Can you work these out from the model? Positions are in its coordinate system, mm. Face numbers are marked on the shaded views. A direction names the side the tool comes from. Round coordinates to 2 decimals unless told otherwise and drop trailing zeros. Write each loop counter-clockwise with the first axis right and the second up, starting at its lowest first coordinate (ties: lowest second). Pieces come first, ordered by that corner, then holes. Notation, with made-up numbers: (-29.75, 51.5) -> (15.25, 51.5) arc R34 ccw to (15.25, 81.5) -> close; hole circle Ø6 at (-10, 7). An arc over 180 degrees is marked (long way). Write item = value, one per line. Start each with the question number.
1) Imagine slicing it at B-B, the plane x = 9. Please give me the cut outline in (y, z), then the cut area to 3 significant figures.
2) I'm going to push flat-ended pins straight in: pin 1 (4 mm diameter, centred on x = -4.5, z = -7.79, fed in from +Y); pin 2 (6 mm diameter, centred on x = 4.5, z = 7.79, fed in from -Y); pin 3 (1 mm diameter, centred on x = 2.5, y = 1.5, fed in from +Z); pin 4 (1.5 mm diameter, centred on y = 3.5, z = -3, fed in from -X). Where does each tip first touch, or does it pass through?
3) Imagine slicing it at A-A, the plane z = 0. Please give me the cut outline in (x, y), then the cut area to 3 significant figures.
4) For the marked faces 1 and 2, which set-ups out of +Z, -Z, +X, -X, +Y, -Y let a thin tool reach every point of the face, with its end or its side?
5) Imagine slicing it at C-C, the plane x = -5. Please give me the cut outline in (y, z).
6) Imagine slicing it at D-D, the plane y = 2.95. Please give me the cut outline in (x, z).
7) Thinking about a two-plate mould opening in Z: for the marked faces 3, 4 and 5, which applies, +Z half, -Z half, draft (parallel to the pull), parting line (faces both ways), or undercut?
8) If I drill on line 1 (X direction, y = 2.8, z = 0); line 2 (Z direction, x = -4.5, y = 3.2); line 3 (X direction, y = 2.9, z = -2.25), over which ranges is the centre line in solid material (lowest first)?
from build123d import *

# Parameters (mm, degrees)
SKETCH_1_R          = 14
EXTRUDE_1_DEPTH     = 2
SKETCH_2_R          = 12.5
EXTRUDE_2_DEPTH     = 3
SKETCH_3_R          = 1.6
CUT_EXTRUDE_1_DEPTH = 6
SKETCH_4_R          = 3
CUT_EXTRUDE_2_DEPTH = 3.3
SKETCH_5_R          = 1.95
CUT_EXTRUDE_3_DEPTH = 3.2
CHAMFER_1_SIZE      = 0.5
SKETCH_6_R          = 3.5
CUT_EXTRUDE_4_DEPTH = 6


with BuildPart() as part:
    # 草图1 → 凸台-拉伸1 (new body)
    with BuildSketch(Plane(origin=(0, 0, 0), x_dir=(1, 0, 0), z_dir=(0, 1, 0))):
        Circle(SKETCH_1_R)
    extrude(amount=EXTRUDE_1_DEPTH)

    # 草图2 → 凸台-拉伸2 (add)
    with BuildSketch(Plane(origin=(0, 2, 0), x_dir=(1, 0, 0), z_dir=(0, 1, 0))):
        Circle(SKETCH_2_R)
    extrude(amount=EXTRUDE_2_DEPTH)

    # 草图3 → 切除-拉伸1 (cut, through all)
    with BuildSketch(Plane(origin=(0, 5, 0), x_dir=(1, 0, 0), z_dir=(0, 1, 0))):
        with Locations((9, 0)):
            Circle(SKETCH_3_R)
        with Locations((-4.5, -7.794228634)):
            Circle(SKETCH_3_R)
        with Locations((-4.5, 7.794228634)):
            Circle(SKETCH_3_R)
    extrude(amount=-CUT_EXTRUDE_1_DEPTH, mode=Mode.SUBTRACT)

    # 草图4 → 切除-拉伸2 (cut)
    with BuildSketch(Plane(origin=(0, 5, 0), x_dir=(1, 0, 0), z_dir=(0, 1, 0))):
        with Locations((9, 0)):
            Circle(SKETCH_4_R)
        with Locations((-4.5, 7.794228634)):
            Circle(SKETCH_4_R)
        with Locations((-4.5, -7.794228634)):
            Circle(SKETCH_4_R)
    extrude(amount=-CUT_EXTRUDE_2_DEPTH, mode=Mode.SUBTRACT)

    # 草图5 → 切除-拉伸3 (cut)
    with BuildSketch(Plane(origin=(0, 5, 0), x_dir=(1, 0, 0), z_dir=(0, 1, 0))):
        with Locations((4.5, 7.794228634)):
            Circle(SKETCH_5_R)
        with Locations((4.5, -7.794228634)):
            Circle(SKETCH_5_R)
        with Locations((-9, 0)):
            Circle(SKETCH_5_R)
    extrude(amount=-CUT_EXTRUDE_3_DEPTH, mode=Mode.SUBTRACT)

    # 倒角1
    chamfer_1_edges = [part.edges().sort_by_distance(p)[0] for p in [
        (2.55, 5, -7.794228634),
        (2.55, 5, 7.794228634),
        (-10.95, 5, 0),
    ]]
    chamfer(chamfer_1_edges, length=CHAMFER_1_SIZE)

    # 草图6 → 切除-拉伸4 (cut, through all)
    with BuildSketch(Plane(origin=(0, 5, 0), x_dir=(1, 0, 0), z_dir=(0, 1, 0))):
        Circle(SKETCH_6_R)
    extrude(amount=-CUT_EXTRUDE_4_DEPTH, mode=Mode.SUBTRACT)


solid = part.part
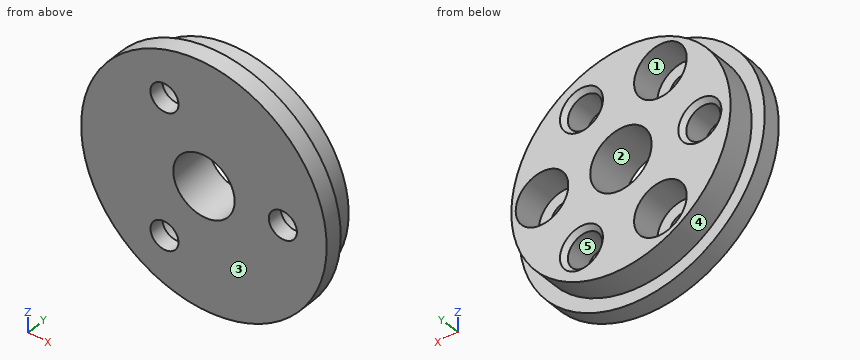
Reported:
q1.outline = (0, -10.72) -> (2, -10.72) -> (2, -8.67) -> (5, -8.67) -> (5, -3) -> (1.7, -3) -> (1.7, -1.6) -> (0, -1.6) -> close; (0, 1.6) -> (1.7, 1.6) -> (1.7, 3) -> (5, 3) -> (5, 8.67) -> (2, 8.67) -> (2, 10.72) -> (0, 10.72) -> close
q1.area = 69.7 mm²
q2.pin_1 = 1.7
q2.pin_2 = 0
q2.pin_3 = 13.86
q2.pin_4 = -12.3
q3.outline = (-14, 0) -> (-3.5, 0) -> (-3.5, 5) -> (-6.55, 5) -> (-7.05, 4.5) -> (-7.05, 1.8) -> (-10.95, 1.8) -> (-10.95, 4.5) -> (-11.45, 5) -> (-12.5, 5) -> (-12.5, 2) -> (-14, 2) -> close; (3.5, 0) -> (7.4, 0) -> (7.4, 1.7) -> (6, 1.7) -> (6, 5) -> (3.5, 5) -> close; (10.6, 0) -> (14, 0) -> (14, 2) -> (12.5, 2) -> (12.5, 5) -> (12, 5) -> (12, 1.7) -> (10.6, 1.7) -> close
q3.area = 58.0 mm²
q4.face_1 = +Y
q4.face_2 = +Y, -Y
q5.outline = (0, -13.08) -> (2, -13.08) -> (2, -11.46) -> (5, -11.46) -> (5, -10.75) -> (1.7, -10.75) -> (1.7, -9.31) -> (0, -9.31) -> close; (0, -6.27) -> (1.7, -6.27) -> (1.7, -4.84) -> (5, -4.84) -> (5, 4.84) -> (1.7, 4.84) -> (1.7, 6.27) -> (0, 6.27) -> close; (0, 9.31) -> (1.7, 9.31) -> (1.7, 10.75) -> (5, 10.75) -> (5, 11.46) -> (2, 11.46) -> (2, 13.08) -> (0, 13.08) -> close
q6.outline = circle Ø25 at (0, 0); hole circle Ø3.9 at (-9, 0); hole circle Ø6 at (-4.5, -7.79); hole circle Ø6 at (-4.5, 7.79); hole circle Ø7 at (0, 0); hole circle Ø3.9 at (4.5, -7.79); hole circle Ø3.9 at (4.5, 7.79); hole circle Ø6 at (9, 0)
q7.face_3 = draft
q7.face_4 = parting line
q7.face_5 = undercut
q8.line_1 = -12.5 to -10.95, -7.05 to -3.5, 3.5 to 6, 12 to 12.5
q8.line_2 = -11.66 to -10.79, -4.79 to 4.79, 10.79 to 11.66
q8.line_3 = -12.3 to -2.68, 2.68 to 7.02, 10.98 to 12.3
